Part model, mm, in its own coordinate system. A direction names the side the tool comes from. Coordinates: 2 decimals unless noted, no trailing zeros. Loops run counter-clockwise (first coordinate to the right, second up) from the corner with the lowest first, then second, coordinate; pieces in that order, holes last. Notation, with made-up numbers: M -28.75,-1.75 L -4.75,-1.75 A9 cw -4.75,7.25 Z; hole C -19,72.25 d9. An arc over 180 degrees is marked long. Answer as a JSON object with one key per item and string values. Group by question number.
1. Saw through at B-B on z = -1.5. Write the cut outline in (x, y), then the cut area to 3 significant figures.
2. Mould opens along X. For faces 1 (the face through (2.44, 0.54, 24.6)), 2 (the face through (-3, 0, -32)), 3 (the face through (11.923, 3.755, 0.434)) say: released by +X, released by -X, zero draft, split by the parting line, or undercut.
3. Drill centre lines: L1, parallel to Y at x = 0, z = -20.25; L2, parallel to X at y = 1, z = 22; L3, parallel to Y at x = 0.5, z = -11. Where is each one in solid material? Low to high.
4. 3-axis set-ups, long thin cutter, end or side, ignore diameter. For faces 4 (the face through (0.424, 0.094, 15.759)), 5 (the face through (2.44, 0.54, -24.6)): which of +Z, -Z, +X, -X, +Y, -Y reach the whole face in a straight line?
5. Drop flat-ended pins along their axis: pin 1 Ø2 at (y, z) = (-4.5, -12.5) entering from -X; pin 2 Ø3 at (x, y) = (0, 0) entering from -Z; pin 3 Ø8 at (x, z) = (7, -14) entering from +Y. Give the stop position or say it passes through.
6. Saw through at A-A on z = 23. Write the cut outline in (x, y).
from build123d import *

# Parameters (mm, degrees)
SKETCH1_R           = 12.5
BOSS_EXTRUDE1_DEPTH = 32
CHAMFER1_SIZE       = 1


with BuildPart() as part:
    # Sketch1 → Boss-Extrude1 (new body, symmetric)
    with BuildSketch(Plane.XY):
        Circle(SKETCH1_R)
    extrude(amount=BOSS_EXTRUDE1_DEPTH, both=True)

    # Chamfer1
    chamfer1_edges = [part.edges().sort_by_distance(p)[0] for p in [
        (-12.5, 0, -32),
        (-12.5, 0, 32),
    ]]
    chamfer(chamfer1_edges, length=CHAMFER1_SIZE)

    # Sketch4 → M6 Tapped Hole1 (revolve, cut)
    with BuildSketch(Plane(origin=(0, 0, 32), x_dir=(0, -1, 0), z_dir=(1, 0, 0))):
        Polygon((0, 0), (0, 16.502151548), (2.5, 15), (2.5, 0), align=None)
    m6_tapped_hole1 = revolve(axis=Axis((0, 0, 38.35), (0, 0, -1)), mode=Mode.SUBTRACT)

    # Mirror1: M6 Tapped Hole1 across plane
    add(m6_tapped_hole1.mirror(Plane.XY), mode=Mode.SUBTRACT)


solid = part.part
Outcome:
{
 "1": {"outline": "C 0,0 d25", "area": "491 mm²"},
 "2": {"face 1": "undercut", "face 2": "zero draft", "face 3": "split by the parting line"},
 "3": {"L1": "y = -12.5 to -2.5, 2.5 to 12.5", "L2": "x = -12.46 to -2.29, 2.29 to 12.46", "L3": "y = -12.49 to 12.49"},
 "4": {"face 4": "+Z", "face 5": "-Z"},
 "5": {"pin 1": "stops at x = -12", "pin 2": "stops at z = -16.4", "pin 3": "stops at y = 12.13"},
 "6": {"outline": "C 0,0 d25; hole C 0,0 d5"}
}
